from build123d import *

# Parameters (mm, degrees)
F1_DEPTH      = 50.8
F2_R          = 12.7
F3_R          = 3.429
F3_R_2        = 17.4625
F4_DEPTH      = 25.4
F4_DEPTH_BACK = 25.4
F5_R          = 1.75
F6_DEPTH      = 89.409


with BuildPart() as f1:
    # F0 (on Front) → F1 (new body)
    with BuildSketch(Plane.XZ):
        Polygon((34.4563108511, 22.225), (-16.8516891489, 22.225), (-16.8516891489, 12.7), (-54.9516891489, 12.7), (-54.9516891489, 0), (72.5563108511, 0), (72.5563108511, 12.7), (34.4563108511, 12.7), align=None)
    extrude(amount=F1_DEPTH)

    # F2
    f2_edges = [f1.edges().sort_by_distance(p)[0] for p in [
        (72.556311, -50.8, 6.35),
        (72.556311, 0, 6.35),
        (-54.951689, -50.8, 6.35),
        (-54.951689, 0, 6.35),
    ]]
    fillet(f2_edges, radius=F2_R)

    # F3 (on face) → F4 (cut, two sides)
    with BuildSketch(Plane.XY.offset(12.7)) as f4_sk:
        with Locations((-42.2516891489, -12.7)):
            Circle(F3_R)
        with Locations((8.8023108511, -25.4)):
            Circle(F3_R_2)
        with Locations((59.8563108511, -38.1)):
            Circle(F3_R)
        with Locations((-42.3004887998, -37.9724390805)):
            Circle(F3_R)
        with Locations((59.8563108511, -12.7)):
            Circle(F3_R)
    extrude(amount=-F4_DEPTH, mode=Mode.SUBTRACT)
    extrude(f4_sk.sketch, amount=F4_DEPTH_BACK, mode=Mode.SUBTRACT)

    # F5 (on face) → F6 (cut, through all)
    with BuildSketch(Plane.YZ.offset(34.4563108511)):
        with Locations((-46.0375, 17.4625)):
            Circle(F5_R)
        with Locations((-4.7625, 17.4625)):
            Circle(F5_R)
    extrude(amount=-F6_DEPTH, mode=Mode.SUBTRACT)


solid = f1.part
Verification items for the finished model (mm, model axes). A direction names the side the tool comes from. Round coordinates to 2 decimals unless told otherwise and drop trailing zeros. Order: outer loops, then holes, each group sorted by start corner. A loop starts at its lowest first (then second) coordinate and runs counter-clockwise, first axis right, second up.
1. Section check A-A on y = -25.4. Record the cut outline in (x, z) (3 decimals), then the cut area to 3 significant figures.
Final values:
outline: (-54.952, 0) - (-8.66, 0) - (-8.66, 22.225) - (-16.852, 22.225) - (-16.852, 12.7) - (-54.952, 12.7) - close; (26.265, 0) - (72.556, 0) - (72.556, 12.7) - (34.456, 12.7) - (34.456, 22.225) - (26.265, 22.225) - close
area: 1,330 mm2
2. Release check for a two-part mould opening along Z. For faces 1 (the flat face through (72.556, -25, 6)), 2 (the flat face through (15, -8, 22.225)), 3 (the cylindrical face through (9, -47, 16)), 4 (the cylindrical face through (9.161, -5.142, 15.754)) record: +Z half, -Z half, draft (parallel to the pull), parting line (faces both ways), or undercut.
Final values:
face 1: draft
face 2: +Z half
face 3: undercut
face 4: undercut
3. Section check B-B on x = 23.5. State how many separate pieces and enclosed holes the cut face has, then the cut area to 3 significant figures.
Final values:
separate pieces: 2
enclosed holes: 2
area: 691 mm2
4. Go/stop test with flat-tipped pins: P1, Ø8, axis at y = -26, z = 19.5, coming from the +X side; P2, Ø8, axis at x = -42.3, y = -37.97, coming from the +Z side; P3, Ø5, axis at y = -14.5, z = 19, coming from the -X side. Record where each tip stops, or that it passes through.
Final values:
P1: stops at x = 34.46
P2: stops at z = 12.7
P3: stops at x = -16.85
5. Thickness scan on L1, parallel to Y at x = -3.5, z = 17.5; L2, parallel to X at y = -25.4, z = 13.25; L3, parallel to Y at x = -45, z = 6.25. Record the ranges inside material, lowest first.
Final values:
L1: y = -50.8 to -47.79, -44.29 to -37.79, -13.01 to -6.51, -3.01 to 0
L2: x = -16.85 to -8.66, 26.26 to 34.46
L3: y = -50.5 to -40.09, -35.86 to -14.75, -10.65 to -0.3
6. Section check D-D on z = 8.25. Record the cut outline in (x, y) (1 decimal), then the cut area to 3 significant figures.
Final values:
outline: (-55, -38.1) arc R12.7 ccw to (-42.3, -50.8) - (59.9, -50.8) arc R12.7 ccw to (72.6, -38.1) - (72.6, -12.7) arc R12.7 ccw to (59.9, 0) - (-42.3, 0) arc R12.7 ccw to (-55, -12.7) - close; hole circle Ø6.9 at (-42.3, -38); hole circle Ø6.9 at (-42.3, -12.7); hole circle Ø34.9 at (8.8, -25.4); hole circle Ø6.9 at (59.9, -38.1); hole circle Ø6.9 at (59.9, -12.7)
area: 5,230 mm2
7. Section check C-C on x = -41. Record the cut outline in (y, z).
Final values:
outline: (-50.8, 0) - (-41.15, 0) - (-41.15, 12.7) - (-50.8, 12.7) - close; (-34.8, 0) - (-15.89, 0) - (-15.89, 12.7) - (-34.8, 12.7) - close; (-9.51, 0) - (0, 0) - (0, 12.7) - (-9.51, 12.7) - close
8. Access from +Z, -Z, +X, -X, +Y, -Y to the whole of each face (thin tool, end or side, straight path). Record for faces 5 (the cylindrical face through (68.935, -46.981, 6.439)), 6 (the flat face through (34.456, -25, 17)), 7 (the flat face through (-36, -25, 12.7)).
Final values:
face 5: +Z, -Z, +X, -Y
face 6: +Z, +X, +Y, -Y
face 7: +Z, -X, +Y, -Y
